Design review of the part built by this model. Coordinates are the model's own, in mm. A direction names the side the tool comes from. Coordinates: 2 decimals unless noted, no trailing zeros. Loops run counter-clockwise (first coordinate to the right, second up) from the corner with the lowest first, then second, coordinate; pieces in that order, holes last. Notation, with made-up numbers: (49, 38.5) - (97, 38.5) arc R10 ccw to (97, 52.5) - close; hole circle Ø3 at (-24.5, -3.5). An arc over 180 degrees is marked (long way). Return JSON: item names as keys, results as strings. Group by question number.
from build123d import *

# Parameters (mm, degrees)
SKETCH1_ONE_SIDE_W   = 1.7526
SKETCH1_ONE_SIDE_H   = 38.1
SKETCH1_ONE_SIDE_W_2 = 2.8702
SKETCH1_ONE_SIDE_H_2 = 3.5052
SKETCH1_ONE_SIDE_W_3 = 4.7625
SKETCH1_ONE_SIDE_H_3 = 0.762


with BuildPart() as part:
    # Sketch1 one side → Revolve1 (revolve)
    with BuildSketch(Plane(origin=(-24.412739892, 0, -3.433041547), x_dir=(0.13925483139909503, 0, -0.9902565788380351), z_dir=(0.9902565788380351, 0, 0.13925483139909503)), mode=Mode.PRIVATE) as revolve1_sk:
        with Locations((9.484713498, -19.83540516)):
            Rectangle(SKETCH1_ONE_SIDE_W, SKETCH1_ONE_SIDE_H)
        with Locations((8.925913498, -40.63800516)):
            Rectangle(SKETCH1_ONE_SIDE_W_2, SKETCH1_ONE_SIDE_H_2)
        with Locations((7.979763498, -38.50440516)):
            Rectangle(SKETCH1_ONE_SIDE_W_3, SKETCH1_ONE_SIDE_H_3)
    revolve(revolve1_sk.sketch.rotate(Axis((-22.969918704, -42.39060516, -13.693103328), (0, 1, 0)), 188.004728857), axis=Axis((-22.969918704, -42.39060516, -13.693103328), (0, 1, 0)))


solid = part.part
Item 1: For faces 1 (the face through (-23, -0.785, -14)), 2 (the face through (-23.096, -40.613, -10.826)), 3 (the face through (-21, -38.123, -14)), list the 3-axis set-ups (+Z, -Z, +X, -X, +Y, -Y) from which the entire face can be reached by the end or side of a thin tool; tool diameter is ignored.
Item 2: Add section B-B (x = -18.75). State the section outline as (y, z) points.
Item 3: Add section C-C (y = -40). State the section outline as (x, z) points.
Item 4: For P1, Ø1.5, axis at x = -22.5, y = -12.5, coming from the +Z side; P2, Ø4, axis at y = -21.5, z = -16.5, coming from the -X side; P3, Ø1, axis at y = -29, z = -13, coming from the -X side, all flat-tipped, find the tip position at first contact; note any pin that passes through.
Item 5: Add section D-D (z = -15). State the section outline as (x, y) points, then the cut area to 3 significant figures.
Item 6: To check wall thickness, follow line 1 (Y direction, x = -21, z = -16.75); line 2 (Y direction, x = -22.75, z = -11.5); line 3 (X direction, y = -39.5, z = -15.75). State the ranges of each line that lie inside material, in increasing order. Write a range as from..to.
Item 7: Add section A-A (z = -11.5). State the section outline as (x, y) points.
Answers below:
{
 "1": {"face 1": "+Z, -Z, +X, -X, +Y", "face 2": "-Y", "face 3": "+Y"},
 "2": {"outline": "(-38.89, -15.9) - (-38.12, -15.9) - (-38.12, -11.49) - (-38.89, -11.49) - close"},
 "3": {"outline": "circle Ø5.74 at (-22.97, -13.69)"},
 "4": {"P1": "stops at z = -11.94", "P2": "stops at x = -24.53", "P3": "stops at x = -24.71"},
 "5": {"outline": "(-27.55, -38.89) - (-25.53, -38.89) - (-25.53, -42.39) - (-20.41, -42.39) - (-20.41, -38.89) - (-18.39, -38.89) - (-18.39, -38.12) - (-21.8, -38.12) - (-21.8, -0.79) - (-24.14, -0.79) - (-24.14, -38.12) - (-27.55, -38.12) - close", "area": "112 mm^2"},
 "6": {"line 1": "y = -38.89..-38.12", "line 2": "y = -42.39..-38.12", "line 3": "x = -24.97..-20.97"},
 "7": {"outline": "(-27.2, -38.89) - (-24.82, -38.89) - (-24.82, -42.39) - (-21.12, -42.39) - (-21.12, -38.89) - (-18.74, -38.89) - (-18.74, -38.12) - (-27.2, -38.12) - close"}
}
